Part model, mm, in its own coordinate system. A direction names the side the tool comes from. Give positions to 0.01 mm unless a question says otherwise; leave off trailing zeros. Order: outer loops, then holes, each group sorted by start corner. A loop starts at its lowest first (then second) coordinate and runs counter-clockwise, first axis right, second up.
1. Mould opens along Z. For faces 3 (the flat face through (-15, 10, -36)), 4 (the flat face through (-14, 10, -41)), 5 (the flat face through (-16, 10, 36)), 6 (the cylindrical face through (-46.022, 10.133, 38.535)) say: +Z half, -Z half, draft (parallel to the pull), parting line (faces both ways), or undercut.
2. Slice it at D-D on y = 15.5. List the corners of the cut face in (x, z), and give its area (3 significant figures).
3. Slice it at C-C on x = -43. List the corners of the cut face in (y, z) (3 decimals), and give its area (4 significant figures).
4. Drop a flat-ended pin along its axis: pin 1 Ø10 at (y, z) = (7, -11) entering from -X. Give the stop position or say it passes through.
5. Probe line 1 (Y direction, x = -43, z = 38) (3 decimals); line 2 (X direction, y = 10, z = -39.8) (3 decimals); line 3 (Z direction, x = -45, y = 3.5). List the from-to ranges inside material, lowest first.
6. Slice it at A-A on y = 10. List the corners of the cut face in (x, z) (3 decimals).
7. Slice it at B-B on x = -8. List the corners of the cut face in (y, z), and give its area (3 significant figures).
8. Which spindle directions (+Z, -Z, +X, -X, +Y, -Y) get a long thin tool onto all of the face, cutting with end or side? Do faces 1 (the flat face through (22, 10, 1)), 2 (the flat face through (-12, 10, 41)). Say none if no direction does.
from build123d import *

# Parameters (mm, degrees)
BOSS_EXTRUDE1_DEPTH = 20
SKETCH3_R           = 3.025
CUT_EXTRUDE1_DEPTH  = 77


with BuildPart() as part:
    # Sketch2 → Boss-Extrude1 (new body)
    with BuildSketch(Plane(origin=(0, 0, 0), x_dir=(1, 0, 0), z_dir=(0, 1, 0))):
        Polygon((-53, 41), (27, 41), (27, -41), (-53, -41), (-53, -36), (22, -36), (22, 36), (-53, 36), align=None)
    extrude(amount=BOSS_EXTRUDE1_DEPTH)

    # Sketch3 → Cut-Extrude1 (cut)
    with BuildSketch(Plane.XY.offset(41)):
        with Locations((-43, 10)):
            Circle(SKETCH3_R)
    cut_extrude1 = extrude(amount=-CUT_EXTRUDE1_DEPTH, mode=Mode.SUBTRACT)

    # Mirror1: Cut-Extrude1 across plane
    add(cut_extrude1.mirror(Plane.XY), mode=Mode.SUBTRACT)


solid = part.part
Data:
1. face 3: undercut
1. face 4: -Z half
1. face 5: undercut
1. face 6: draft
2. outline: (-53, -41) - (27, -41) - (27, 41) - (-53, 41) - (-53, 36) - (22, 36) - (22, -36) - (-53, -36) - close
2. area: 1,160 mm2
3. outline: (0, -41) - (6.975, -41) - (6.975, -36) - (0, -36) - close; (0, 36) - (6.975, 36) - (6.975, 41) - (0, 41) - close; (13.025, -41) - (20, -41) - (20, -36) - (13.025, -36) - close; (13.025, 36) - (20, 36) - (20, 41) - (13.025, 41) - close
3. area: 139.5 mm2
4. pin 1: stops at x = 22
5. line 1: y = 0 to 6.975, 13.025 to 20
5. line 2: x = -53 to -46.025, -39.975 to 27
5. line 3: z = -41 to -36, 36 to 41
6. outline: (-53, -41) - (-46.025, -41) - (-46.025, -36) - (-53, -36) - close; (-53, 36) - (-46.025, 36) - (-46.025, 41) - (-53, 41) - close; (-39.975, -41) - (27, -41) - (27, 41) - (-39.975, 41) - (-39.975, 36) - (22, 36) - (22, -36) - (-39.975, -36) - close
7. outline: (0, -41) - (20, -41) - (20, -36) - (0, -36) - close; (0, 36) - (20, 36) - (20, 41) - (0, 41) - close
7. area: 200 mm2
8. face 1: -X, +Y, -Y
8. face 2: +Z, +X, -X, +Y, -Y
